from build123d import *
from build123d.topology import SkipClean

# Parameters (mm, degrees)
SKETCH1_R           = 47.99995
SKETCH1_R_2         = 19.35
SKETCH1_W           = 70
SKETCH1_H           = 6.35
BOSS_EXTRUDE1_DEPTH = 7.5
SKETCH1_3_W         = 70
SKETCH1_3_H         = 6.35
BOSS_EXTRUDE2_DEPTH = 5
SKETCH2_W           = 70
SKETCH2_H           = 6.35
BOSS_EXTRUDE3_DEPTH = 10
SKETCH3_R           = 19.35
BOSS_EXTRUDE4_DEPTH = 15
SKETCH4_R           = 47.99995
SKETCH4_R_2         = 40.49995
BOSS_EXTRUDE5_DEPTH = 7.5


with BuildPart() as part:
    # Sketch1 → Boss-Extrude1 (new body)
    with BuildSketch(Plane(origin=(0, 0, 0), x_dir=(0, 0, -1), z_dir=(1, 0, 0))):
        Circle(SKETCH1_R)
        with Locations((0, -16.134793457)):
            Circle(SKETCH1_R_2, mode=Mode.SUBTRACT)
        with Locations((0, 9.390206543)):
            Rectangle(SKETCH1_W, SKETCH1_H, mode=Mode.SUBTRACT)
    extrude(amount=-BOSS_EXTRUDE1_DEPTH)

    # Sketch1<3> → Boss-Extrude2 (add)
    with BuildSketch(Plane(origin=(0, 0, 0), x_dir=(0, 0, -1), z_dir=(1, 0, 0))):
        with Locations((0, 9.390206543)):
            Rectangle(SKETCH1_3_W, SKETCH1_3_H)
    extrude(amount=-BOSS_EXTRUDE2_DEPTH)

    # Sketch2 → Boss-Extrude3 (add)
    with SkipClean():  # the faces are left unmerged after this step: merging them gives an invalid solid
        with BuildSketch(Plane.ZY.offset(7.5)):
            with BuildLine():
                Line((-47.443323347, -7.288776975), (-36.939339828, 3.215206543))
                Line((-36.939339828, 3.215206543), (36.939339828, 3.215206543))
                Line((36.939339828, 3.215206543), (47.443323347, -7.288776975))
                ThreePointArc((47.443323347, -7.288776975), (47.577493547, -6.354314108), (47.693260005, -5.41739329))
                Line((47.693260005, -5.41739329), (38, 4.275866715))
                Line((38, 4.275866715), (38, 14.504546372))
                Line((38, 14.504546372), (43.590913129, 20.095459501))
                ThreePointArc((43.590913129, 20.095459501), (43.252246865, 20.814378231), (42.901724899, 21.527591614))
                Line((42.901724899, 21.527591614), (36.939339828, 15.565206543))
                Line((36.939339828, 15.565206543), (-36.939339828, 15.565206543))
                Line((-36.939339828, 15.565206543), (-42.901724899, 21.527591614))
                ThreePointArc((-42.901724899, 21.527591614), (-43.252246865, 20.814378231), (-43.590913129, 20.095459501))
                Line((-43.590913129, 20.095459501), (-38, 14.504546372))
                Line((-38, 14.504546372), (-38, 4.275866715))
                Line((-38, 4.275866715), (-47.693260005, -5.41739329))
                ThreePointArc((-47.693260005, -5.41739329), (-47.577493547, -6.354314108), (-47.443323347, -7.288776975))
            make_face()
            with Locations((0, 9.390206543)):
                Rectangle(SKETCH2_W, SKETCH2_H, mode=Mode.SUBTRACT)
        extrude(amount=BOSS_EXTRUDE3_DEPTH)

    # Sketch3 → Boss-Extrude4 (add)
    with SkipClean():  # the faces are left unmerged after this step: merging them gives an invalid solid
        with BuildSketch(Plane.ZY.offset(7.5)):
            with BuildLine():
                Line((14.879516121, 6.215206543), (-14.879516121, 6.215206543))
                ThreePointArc((-14.879516121, 6.215206543), (0, -42.984793457), (14.879516121, 6.215206543))
            make_face()
            with Locations(Location((0, -16.134793457, 0), (0, 0, 180))):
                Circle(SKETCH3_R, mode=Mode.SUBTRACT)
        extrude(amount=BOSS_EXTRUDE4_DEPTH)

    # Sketch4 → Boss-Extrude5 (add)
    with SkipClean():  # the faces are left unmerged after this step: merging them gives an invalid solid
        with BuildSketch(Plane.ZY.offset(7.5)):
            with Locations(Location((0, 0, 0), (0, 0, 180))):
                Circle(SKETCH4_R)
            Circle(SKETCH4_R_2, mode=Mode.SUBTRACT)
        extrude(amount=BOSS_EXTRUDE5_DEPTH)


solid = part.part
The listing builds one solid part. Answer for the finished solid, in the listing's coordinates (mm). A direction names the side the tool comes from. Give positions to 0.01 mm unless a question says otherwise; leave off trailing zeros. Write each loop counter-clockwise with the first axis right and the second up, starting at its lowest first coordinate (ties: lowest second). Pieces come first, ordered by that corner, then holes.
1) Section B-B (y = 33) is taken. Write down the section's boundary in (x, z), and give its area (3 significant figures).
2) A tool of negligible diameter and unlimited length cuts with its end or side. For faces 4 (the face through (-13.541, 0.224, -39.931)), 5 (the face through (-15, -44, 0)), 6 (the face through (-22.5, -24, -18)), from which of +Z, -Z, +X, -X, +Y, -Y can it reach the whole face along a straight path? Write none if from no direction.
3) For a pull along Z with two mould halves and no side action, classify faces 1 (the face through (-15, 7, -44)), 2 (the face through (-15.763, 1.515, 40.76)), 3 (the face through (-11.2, -21.49, -34.33)) as pulls with the +Z half, pulls with the -Z half, needs draft (parallel to the pull), parting line crosses it, or undercut.
4) Section D-D (y = -8.5) is taken. Write down the section's boundary in (x, z).
5) Section C-C (x = -11) is taken. Write down the section's boundary in (y, z).
6) Find the intervals of material crossed by L1, parallel to Y at x = -11.75, z = 0; L2, parallel to Z at x = -14, y = 4; L3, parallel to Y at x = -15.25, z = -14, in increasing order.
7) Section A-A (z = 0) is taken. Write down the section's boundary in (x, y).
8) Given P1, Ø12, axis at y = 13, z = -19, coming from the +X side; P2, Ø5, axis at x = -15, z = -23.5, coming from the -Y side; P3, Ø4, axis at x = -10.5, z = -18.5, coming from the -Y side; P4, Ø11, axis at x = -10, y = 9, coming from the +Z side, each flat-ended and moving along its own axis, determine where each tip first touches the part or whether it passes through.
Response:
1. outline: (-15, -34.86) - (0, -34.86) - (0, 34.86) - (-15, 34.86) - (-15, 23.48) - (-7.5, 23.48) - (-7.5, -23.48) - (-15, -23.48) - close
1. area: 694 mm2
2. face 4: -X
2. face 5: -X, -Y
2. face 6: +Z, -Z, -X, +Y, -Y
3. face 1: needs draft
3. face 2: undercut
3. face 3: undercut
4. outline: (-22.5, -25.74) - (-7.5, -25.74) - (-7.5, -39.6) - (-15, -39.6) - (-15, -47.24) - (0, -47.24) - (0, -17.78) - (-22.5, -17.78) - close; (-22.5, 17.78) - (0, 17.78) - (0, 47.24) - (-15, 47.24) - (-15, 39.6) - (-7.5, 39.6) - (-7.5, 25.74) - (-22.5, 25.74) - close
5. outline: (20.1, -43.59) arc R48 ccw to (21.53, -42.9) arc R48 ccw to (21.53, 42.9) arc R48 ccw to (20.1, 43.59) arc R48 ccw (long way) to start; hole (-36.56, -17.43) arc R40.5 ccw to (-0.34, -40.5) - (3.22, -36.94) - (3.22, -18.61) arc R26.85 cw to start; hole (-36.56, 17.43) arc R26.85 cw to (3.22, 18.61) - (3.22, 36.94) - (-0.34, 40.5) arc R40.5 ccw to start; hole circle Ø38.7 at (-16.13, 0); hole (1.82, -40.46) arc R40.5 ccw to (14.01, -38) - (4.28, -38) - close; hole (1.82, 40.46) - (4.28, 38) - (14.01, 38) arc R40.5 ccw to start; hole (6.22, -35) - (12.57, -35) - (12.57, 35) - (6.22, 35) - close; hole (15.57, -36.94) - (15.88, -37.26) arc R40.5 ccw to (15.88, 37.26) - (15.57, 36.94) - close
6. L1: y = -48 to -35.48, 3.22 to 6.22, 12.57 to 15.57, 40.5 to 48
6. L2: z = -47.83 to -40.3, -38.28 to 38.28, 40.3 to 47.83
6. L3: y = -39.05 to -29.49, -2.78 to 6.22, 12.57 to 15.57
7. outline: (-22.5, -42.98) - (-15, -42.98) - (-15, -48) - (0, -48) - (0, -35.48) - (-22.5, -35.48) - close; (-22.5, 3.22) - (0, 3.22) - (0, 48) - (-15, 48) - (-15, 40.5) - (-7.5, 40.5) - (-7.5, 15.57) - (-17.5, 15.57) - (-17.5, 12.57) - (-5, 12.57) - (-5, 6.22) - (-22.5, 6.22) - close
8. P1: stops at x = 0
8. P2: stops at y = -43.16
8. P3: stops at y = -45.07
8. P4: stops at z = 47.87
